```python
from build123d import *

# Parameters (mm, degrees)
SKETCH_1_R                  = 7.4
EXTRUDE_1_DEPTH             = 5
SKETCH_2_R                  = 8.9
EXTRUDE_2_DEPTH             = 1
SKETCH_3_R                  = 15
EXTRUDE_3_DEPTH             = 20
SKETCH_11_W                 = 20
SKETCH_11_H                 = 20
EXTRUDE_8_DEPTH             = 40
EXTRUDE_4_DEPTH             = 20
EXTRUDE_START               = 9
SKETCH_5_R                  = 7
EXTRUDE_5_DEPTH             = 9
HOLE_WIZARD_M51_D           = 5.5
HOLE_WIZARD_M51_CBORE_D     = 10.5
HOLE_WIZARD_M51_CBORE_DEPTH = 14
CHAMFER_1_SIZE              = 3
FILLET_20_R                 = 40
SKETCH_8_R                  = 9
EXTRUDE_6_DEPTH             = 1
SKETCH_9_R                  = 7.5
EXTRUDE_7_DEPTH             = 5
SKETCH_13_W                 = 34
SKETCH_13_H                 = 20
EXTRUDE_9_DEPTH             = 12
SKETCH_14_R                 = 7.2
CUT_EXTRUDE_3_DEPTH         = 45
SKETCH_15_W                 = 34
SKETCH_15_H                 = 3
CUT_EXTRUDE_4_DEPTH         = 25
CUT_EXTRUDE_5_DEPTH         = 52.166395
CUT_EXTRUDE_5_DEPTH_BACK    = 52.166395
FILLET_14_R                 = 1
CUT_EXTRUDE_6_DEPTH         = 14
CUT_EXTRUDE_7_DEPTH         = 64.584589
SKETCH_19_W                 = 5.4
SKETCH_19_H                 = 10.4
CUT_EXTRUDE_8_DEPTH         = 5
FILLET_15_R                 = 1
FILLET_18_R                 = 0.4
HOLE_WIZARD_M41_D           = 4.5
FILLET_19_R                 = 6
FILLET_21_R                 = 3


with BuildPart() as part:
    # Эскиз1 → Бобышка-Вытянуть1 (new body)
    with BuildSketch(Plane.XY):
        Circle(SKETCH_1_R)
    extrude(amount=EXTRUDE_1_DEPTH)

    # Эскиз2 → Бобышка-Вытянуть2 (add)
    with BuildSketch(Plane(origin=(0, 0, 0), x_dir=(-1, 0, 0), z_dir=(0, 0, -1))):
        Circle(SKETCH_2_R)
    extrude(amount=EXTRUDE_2_DEPTH)

    # Эскиз3 → Бобышка-Вытянуть3 (add)
    with BuildSketch(Plane(origin=(0, 0, -1), x_dir=(-1, 0, 0), z_dir=(0, 0, -1))):
        Circle(SKETCH_3_R)
    extrude(amount=EXTRUDE_3_DEPTH)

    # Эскиз11 → Бобышка-Вытянуть8 (add)
    with BuildSketch(Plane(origin=(0, 0, 0), x_dir=(1, 0, 0), z_dir=(0, 1, 0))):
        with Locations((0, 11)):
            Rectangle(SKETCH_11_W, SKETCH_11_H)
    extrude(amount=-EXTRUDE_8_DEPTH)

    # Эскиз4 → Бобышка-Вытянуть4 (add)
    with BuildSketch(Plane(origin=(0, 0, -1), x_dir=(-1, 0, 0), z_dir=(0, 0, -1))):
        with BuildLine():
            Line((-6.631923, 27.24), (-14.211263, 4.8))
            Line((-14.211263, 4.8), (14.211263, 4.8))
            Line((14.211263, 4.8), (6.631923, 27.24))
            ThreePointArc((6.631923, 27.24), (0, 32), (-6.631923, 27.24))
        make_face()
    extrude(amount=EXTRUDE_4_DEPTH)

    # Эскиз5 → Бобышка-Вытянуть5 (add)
    with BuildSketch(Plane.XY.offset(-1).offset(EXTRUDE_START)):
        with Locations((0, 25)):
            Circle(SKETCH_5_R)
    extrude(amount=-EXTRUDE_5_DEPTH)

    # Цековка для винта с внутренним шестигранником M51 (through all)
    with Locations(Plane(origin=(0.481722, 0.624121, -21), x_dir=(-1, 0, 0), z_dir=(0, 0, -1))):
        with Locations((0.481722, 24.375879)):
            CounterBoreHole(HOLE_WIZARD_M51_D / 2, HOLE_WIZARD_M51_CBORE_D / 2, HOLE_WIZARD_M51_CBORE_DEPTH)

    # Фаска1
    chamfer_1_edges = [part.edges().sort_by_distance(p)[0] for p in [
        (-7, 25, 8),
    ]]
    chamfer(chamfer_1_edges, length=CHAMFER_1_SIZE)

    # Скругление20
    fillet_20_edges = [part.edges().sort_by_distance(p)[0] for p in [
        (10, -11.18034, -11),
        (-10, -11.18034, -11),
    ]]
    fillet(fillet_20_edges, radius=FILLET_20_R)

    # Эскиз8 → Бобышка-Вытянуть6 (add)
    with BuildSketch(Plane(origin=(0, 0, -21), x_dir=(-1, 0, 0), z_dir=(0, 0, -1))):
        Circle(SKETCH_8_R)
    extrude(amount=EXTRUDE_6_DEPTH)

    # Эскиз9 → Бобышка-Вытянуть7 (add)
    with BuildSketch(Plane(origin=(0, 0, -22), x_dir=(-1, 0, 0), z_dir=(0, 0, -1))):
        Circle(SKETCH_9_R)
    extrude(amount=EXTRUDE_7_DEPTH)

    # Эскиз13 → Бобышка-Вытянуть9 (add)
    with BuildSketch(Plane(origin=(0, -40, 0), x_dir=(-1, 0, 0), z_dir=(0, -1, 0))):
        with Locations((0, 11)):
            Rectangle(SKETCH_13_W, SKETCH_13_H)
    extrude(amount=-EXTRUDE_9_DEPTH)

    # Эскиз14 → Вырез-Вытянуть3 (cut)
    with BuildSketch(Plane(origin=(0, -40, 0), x_dir=(-1, 0, 0), z_dir=(0, -1, 0))):
        with Locations(Location((0, 11, 0), (0, 0, 90))):
            Circle(SKETCH_14_R)
    extrude(amount=-CUT_EXTRUDE_3_DEPTH, mode=Mode.SUBTRACT)

    # Эскиз15 → Вырез-Вытянуть4 (cut)
    with BuildSketch(Plane(origin=(0, -40, 0), x_dir=(-1, 0, 0), z_dir=(0, -1, 0))):
        with Locations((0, 11)):
            Rectangle(SKETCH_15_W, SKETCH_15_H)
    extrude(amount=-CUT_EXTRUDE_4_DEPTH, mode=Mode.SUBTRACT)

    # Эскиз16 → Вырез-Вытянуть5 (cut, two sides: drawn at the far end of the back side and taken through both)
    with BuildSketch(Plane(origin=(0, 0, 0), x_dir=(0, 0, -1), z_dir=(1, 0, 0)).offset(-CUT_EXTRUDE_5_DEPTH_BACK)):
        with BuildLine():
            Line((9.5, -15), (12.5, -15))
            ThreePointArc((12.5, -15), (11, -13.5), (9.5, -15))
        make_face()
    extrude(amount=CUT_EXTRUDE_5_DEPTH + CUT_EXTRUDE_5_DEPTH_BACK, mode=Mode.SUBTRACT)

    # Скругление14
    fillet_14_edges = [part.edges().sort_by_distance(p)[0] for p in [
        (0, -40, -3.8),
        (-4.529901, -40, -16.596427),
    ]]
    fillet(fillet_14_edges, radius=FILLET_14_R)

    # Эскиз17 → Вырез-Вытянуть6 (cut)
    with BuildSketch(Plane(origin=(0, 0, -21), x_dir=(-1, 0, 0), z_dir=(0, 0, -1))):
        with BuildLine():
            Line((5.25, 25), (5.25, 15))
            ThreePointArc((5.25, 15), (0, 9.75), (-5.25, 15))
            Line((-5.25, 15), (-5.25, 25))
            ThreePointArc((-5.25, 25), (0, 30.25), (5.25, 25))
        make_face()
    extrude(amount=-CUT_EXTRUDE_6_DEPTH, mode=Mode.SUBTRACT)

    # Эскиз18 → Вырез-Вытянуть7 (cut, through all)
    with BuildSketch(Plane(origin=(0, 15, 0), x_dir=(-1, 0, 0), z_dir=(0, -1, 0))):
        with BuildLine():
            Line((-5.25, 7), (5.25, 7))
            Line((5.25, 7), (5.25, 15.92722))
            ThreePointArc((5.25, 15.92722), (0, 18.2), (-5.25, 15.92722))
            Line((-5.25, 15.92722), (-5.25, 7))
        make_face()
    extrude(amount=CUT_EXTRUDE_7_DEPTH, mode=Mode.SUBTRACT)

    # Эскиз19 → Вырез-Вытянуть8 (cut)
    with BuildSketch(Plane(origin=(0, 0, -27), x_dir=(-1, 0, 0), z_dir=(0, 0, -1))):
        Rectangle(SKETCH_19_W, SKETCH_19_H)
    extrude(amount=-CUT_EXTRUDE_8_DEPTH, mode=Mode.SUBTRACT)

    # Скругление15
    fillet_15_edges = [part.edges().sort_by_distance(p)[0] for p in [
        (5.25, 10, -7),
        (-5.25, 10, -7),
        (0, 30.25, -7),
    ]]
    fillet(fillet_15_edges, radius=FILLET_15_R)

    # Скругление18
    fillet_18_edges = [part.edges().sort_by_distance(p)[0] for p in [
        (-2.7, 5.2, -24.5),
        (-2.7, -5.2, -24.5),
        (2.7, -5.2, -24.5),
        (2.7, 5.2, -24.5),
    ]]
    fillet(fillet_18_edges, radius=FILLET_18_R)

    # Отверстие с зазором M41 (through all)
    with Locations(Plane.XY.offset(-1)):
        with Locations((-12, -34), (11, -34)):
            Hole(HOLE_WIZARD_M41_D / 2)

    # Скругление19
    fillet_19_edges = [part.edges().sort_by_distance(p)[0] for p in [
        (17, -28, -16.75),
        (17, -28, -5.25),
        (17, -40, -5.25),
        (17, -40, -16.75),
        (-17, -28, -16.75),
        (-17, -40, -16.75),
        (-17, -28, -5.25),
        (-17, -40, -5.25),
    ]]
    fillet(fillet_19_edges, radius=FILLET_19_R - 0.0001)  # a hair under: the kernel refuses the full size

    # Скругление21
    fillet_21_edges = [part.edges().sort_by_distance(p)[0] for p in [
        (10, -28, -16.75),
        (10, -28, -5.25),
        (-10, -28, -16.75),
        (-10, -28, -5.25),
    ]]
    fillet(fillet_21_edges, radius=FILLET_21_R)


solid = part.part
```
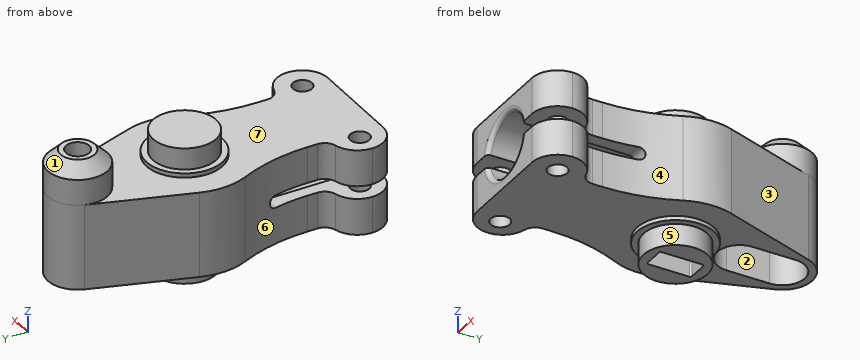
Input: part model. Units: mm. Frame: model coordinates. Face numbers are marked on the shaded views. A direction names the side the tool comes from. Round coordinates to 2 decimals unless told otherwise and drop trailing zeros. Loops run counter-clockwise (first coordinate to the right, second up) from the corner with the lowest first, then second, coordinate; pieces in that order, holes last. Notation, with made-up numbers: (-9, -37.75) -> (20, -37.75) arc R24 cw to (20, -3.75) -> close; hole circle Ø8 at (-35.75, 42). An arc over 180 degrees is marked (long way). One line per item, written item: value.
(1) Mould query, pull axis Y, two halves, no side actions, for the marked faces 1, 2, 3 and 4. Classes: pulls with the +Y half, pulls with the -Y half, needs draft (parallel to the pull), parting line crosses it, or undercut.
Geometry check:
face 1: parting line crosses it
face 2: undercut
face 3: pulls with the +Y half
face 4: undercut
(2) Set-up query: the marked faces 5, 6 and 7. Return all of +Z, -Z, +X, -X, +Y, -Y with unobstructed straight access to the full face (end or side cutting, diameter ignored); none if empty.
Geometry check:
face 5: -Z
face 6: +Z, -Z, -X
face 7: +Z
(3) Section C-C (z = -20). Give the number of separate pieces and of enclosed holes in the cut face, plus the area to 3 significant figures.
Geometry check:
separate pieces: 1
enclosed holes: 3
area: 1,470 mm2
(4) Pin query (flat end, axial travel): pin 1 (4 mm diameter, centred on x = -12, y = -34, fed in from +Z); pin 2 (12 mm diameter, centred on x = -8.5, y = -31.5, fed in from +Z); pin 3 (6 mm diameter, centred on y = -2, z = -10.5, fed in from -X); pin 4 (12 mm diameter, centred on y = -24, z = -12.5, fed in from +X). Return the tip coordinate at first contact, or that it passes through.
Geometry check:
pin 1: through
pin 2: z = -1
pin 3: x = -15
pin 4: x = 15.47
(5) Material intervals for line 1 (Z direction, x = 9, y = -19.5); line 2 (Z direction, x = -3.5, y = -33.5); line 3 (Y direction, x = -4.5, z = 4.5), sorted ascending. Write a range as [from, to].
Geometry check:
line 1: [-21, -12.5], [-9.5, -1]
line 2: [-21, -17.29], [-4.71, -1]
line 3: [-5.87, 5.87], [19.64, 30.36]
(6) Section A-A (y = -30.5). Return the cut outline in (x, z).
Geometry check:
outline: (-15.87, -21) -> (15.87, -21) -> (15.87, -12.5) -> (7.04, -12.5) arc R7.2 cw to (-7.04, -12.5) -> (-15.87, -12.5) -> close; (-15.87, -9.5) -> (-7.04, -9.5) arc R7.2 cw to (7.04, -9.5) -> (15.87, -9.5) -> (15.87, -1) -> (-15.87, -1) -> close
(7) Section B-B (y = 2). Return the cut outline in (x, z).
Geometry check:
outline: (-14.87, -21) -> (-8.77, -21) -> (-8.77, -22) -> (-7.23, -22) -> (-7.23, -27) -> (-2.7, -27) -> (-2.7, -22) -> (2.7, -22) -> (2.7, -27) -> (7.23, -27) -> (7.23, -22) -> (8.77, -22) -> (8.77, -21) -> (14.87, -21) -> (14.87, -1) -> (8.67, -1) -> (8.67, 0) -> (7.12, 0) -> (7.12, 5) -> (-7.12, 5) -> (-7.12, 0) -> (-8.67, 0) -> (-8.67, -1) -> (-14.87, -1) -> close; hole circle Ø14.4 at (0, -11)
